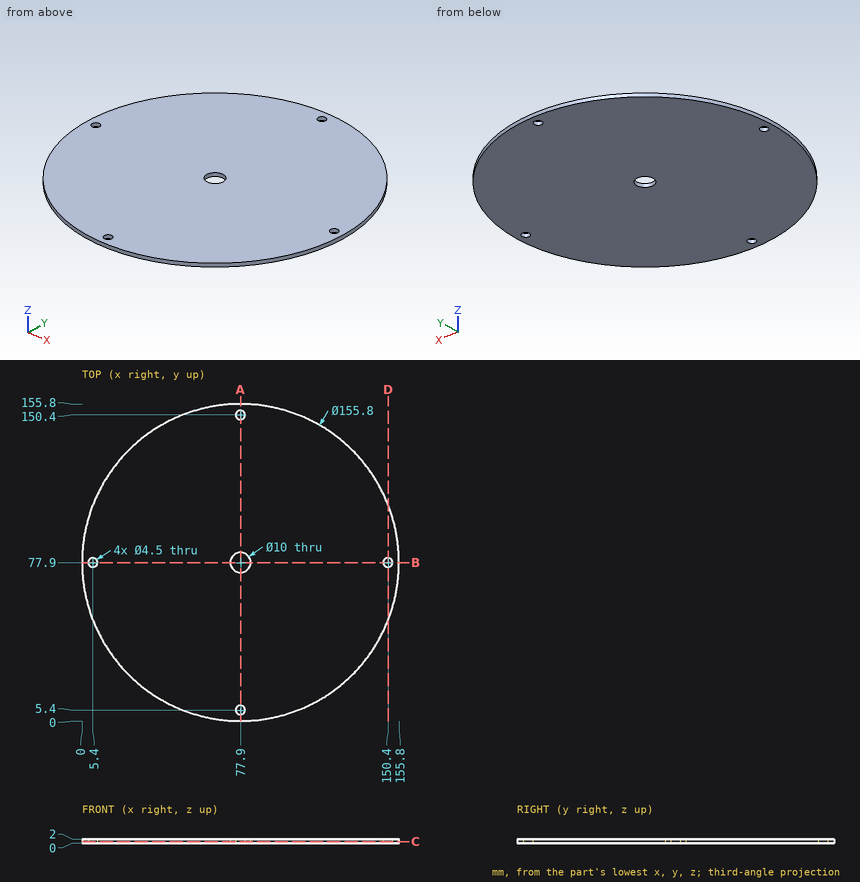
Could you check a few things on this drawing? It's one solid part, dimensions in mm from its lowest x, y, z. Coordinates: 2 decimals unless noted, no trailing zeros. Write each loop counter-clockwise with the first axis right and the second up, starting at its lowest first coordinate (ties: lowest second). Pieces come first, ordered by that corner, then holes. Notation, with made-up numbers: (81, 38) - (140, 38) arc R23 cw to (140, 61) - close; hole circle Ø11 at (86, 88). An arc over 180 degrees is marked (long way). Put each result on its own line as item: value. Start each with the question number.
Q1. Please list where these lines run through material, in increasing order: L1, parallel to Y at x = 77.9, z = 1.05; L2, parallel to X at y = 149, z = 1.2; L3, parallel to Y at x = 28, z = 1.85.
Q2. I want a section at A-A on x = 77.9. Write out the boundary of the cut face in (y, z), plus the area to 3 significant figures.
Q3. I want a section at D-D on x = 150.4. Write out the boundary of the cut face in (y, z).
Q4. I want a section at C-C on z = 0.7. Write out the boundary of the cut face in (x, y).
Checks:
1. L1: 0 to 3.15, 7.65 to 72.9, 82.9 to 148.15, 152.65 to 155.8
1. L2: 46.07 to 76.14, 79.66 to 109.73
1. L3: 18.08 to 137.72
2. outline: (0, 0) - (3.15, 0) - (3.15, 2) - (0, 2) - close; (7.65, 0) - (72.9, 0) - (72.9, 2) - (7.65, 2) - close; (82.9, 0) - (148.15, 0) - (148.15, 2) - (82.9, 2) - close; (152.65, 0) - (155.8, 0) - (155.8, 2) - (152.65, 2) - close
2. area: 274 mm²
3. outline: (49.4, 0) - (75.65, 0) - (75.65, 2) - (49.4, 2) - close; (80.15, 0) - (106.4, 0) - (106.4, 2) - (80.15, 2) - close
4. outline: circle Ø155.8 at (77.9, 77.9); hole circle Ø4.5 at (5.4, 77.9); hole circle Ø10 at (77.9, 77.9); hole circle Ø4.5 at (77.9, 5.4); hole circle Ø4.5 at (77.9, 150.4); hole circle Ø4.5 at (150.4, 77.9)
